```python
from build123d import *

# Parameters (mm, degrees)
F0_R     = 11.1
F1_DEPTH = 7
F2_R     = 7.62
F3_DEPTH = 25.4


with BuildPart() as f1:
    # F0 (on Top) → F1 (new body)
    with BuildSketch(Plane.XY):
        with BuildLine():
            ThreePointArc((0, -11.1), (7.848885, -7.848885), (11.1, 0))
            ThreePointArc((11.1, 0), (-7.848885, 7.848885), (0, -11.1))
        make_face()
        Polygon((-47.625, -27.94), (0, -27.94), (47.625, -27.94), (0, 53.81), align=None)
        with Locations((-22.521795, -13.005035)):
            Circle(F0_R, mode=Mode.SUBTRACT)
        with Locations((22.521795, -13.005035)):
            Circle(F0_R, mode=Mode.SUBTRACT)
        with BuildLine():
            ThreePointArc((0, -11.1), (-7.848885, 7.848885), (11.1, 0))
            ThreePointArc((11.1, 0), (7.848885, -7.848885), (0, -11.1))
        make_face(mode=Mode.SUBTRACT)
        with Locations((0, 25.87)):
            Circle(F0_R, mode=Mode.SUBTRACT)
    extrude(amount=F1_DEPTH)

    # F2 (on face) → F3 (cut)
    with BuildSketch(Plane.XY.offset(7)):
        with Locations((0, -27.94)):
            Circle(F2_R)
        with Locations((24.19675, 13.97)):
            Circle(F2_R)
        with Locations((-24.19675, 13.97)):
            Circle(F2_R)
    extrude(amount=-F3_DEPTH, mode=Mode.SUBTRACT)


solid = f1.part
```
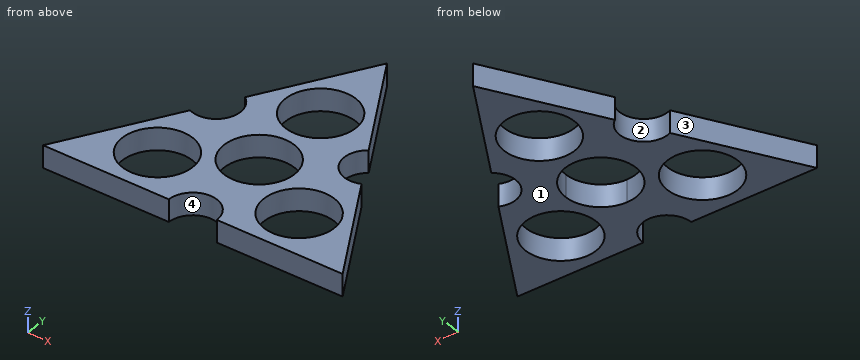
The listing builds one solid part. Answer for the finished solid, in the listing's coordinates (mm). Face numbers are marked on the shaded views. Give positions to 0.01 mm unless a question says otherwise; leave off trailing zeros. Write each loop counter-clockwise with the first axis right and the second up, starting at its lowest first coordinate (ties: lowest second). Pieces come first, ordered by that corner, then holes. Notation, with made-up numbers: (87, -34) -> (146, -34) arc R18 cw to (146, -23) -> close; hole circle Ø2 at (54, -16). An arc over 180 degrees is marked (long way). Write item = value, one per line. Start each with the question number.
1) Each of these flat-tipped pins is pushed along its axis until it touches: pin 1 (4 mm diameter, centred on x = -16.5, z = 3.5, fed in from +Y); pin 2 (1 mm diameter, centred on y = 9.5, z = 4.5, fed in from -X). Where does it stop, or does it pass through?
2) Straight lines are drawn through the part: line 1 along Y through (x, z) = (-18, 5.75); line 2 along X through (y, z) = (-6, 5); line 3 along X through (y, z) = (-14, 6.5). For each, find the intervals that lie inside material, in ascending order.
3) Determine the mould class of the marked faces 1, 2, 3 and 4 for opening direction X: +X half, -X half, draft (parallel to the pull), parting line (faces both ways), or undercut.
4) The part is cut by section C-C, the plane x = 5. Determine the outline of the cut face in (y, z), and give its area (3 significant figures).
5) The part is cut by section A-A, the plane y = 17.5. Determine the outline of the cut face in (x, z), and give its area (3 significant figures).
6) The part is cut by section D-D, the plane y = 25.87. Determine the outline of the cut face in (x, z), and give its area (3 significant figures).
7) The part is cut by section B-B, the plane z = 3.75. Determine the outline of the cut face in (x, y) (3 decimals).
Solutions:
q1.pin_1 = 28.92
q1.pin_2 = -18.42
q2.line_1 = -27.94 to -23.14, -2.87 to 9.54, 18.4 to 22.91
q2.line_2 = -34.84 to -31.13, -13.91 to -9.34, 9.34 to 13.91, 31.13 to 34.84
q2.line_3 = -39.5 to -33.58, -11.47 to 11.47, 33.58 to 39.5
q3.face_1 = draft
q3.face_2 = undercut
q3.face_3 = -X half
q3.face_4 = undercut
q4.outline = (-22.19, 0) -> (-9.91, 0) -> (-9.91, 7) -> (-22.19, 7) -> close; (9.91, 0) -> (15.96, 0) -> (15.96, 7) -> (9.91, 7) -> close; (35.78, 0) -> (45.23, 0) -> (45.23, 7) -> (35.78, 7) -> close
q4.area = 194 mm²
q5.outline = (-17.44, 0) -> (-7.29, 0) -> (-7.29, 7) -> (-17.44, 7) -> close; (7.29, 0) -> (17.44, 0) -> (17.44, 7) -> (7.29, 7) -> close
q5.area = 142 mm²
q6.outline = (-16.28, 0) -> (-11.1, 0) -> (-11.1, 7) -> (-16.28, 7) -> close; (11.1, 0) -> (16.28, 0) -> (16.28, 7) -> (11.1, 7) -> close
q6.area = 72.5 mm²
q7.outline = (-47.625, -27.94) -> (-7.62, -27.94) arc R7.62 cw to (7.62, -27.94) -> (47.625, -27.94) -> (27.271, 6.998) arc R7.62 cw to (19.648, 20.083) -> (0, 53.81) -> (-19.648, 20.083) arc R7.62 cw to (-27.271, 6.998) -> close; hole circle Ø22.2 at (-22.522, -13.005); hole circle Ø22.2 at (0, 25.87); hole (0, -11.1) arc R11.1 ccw to (11.1, 0) arc R11.1 ccw (long way) to start; hole circle Ø22.2 at (22.522, -13.005)
